CAD build for the part. Positions are in the model's coordinates, mm. Face numbers are marked on the shaded views. Round coordinates to 2 decimals unless told otherwise and drop trailing zeros. Loops run counter-clockwise (first coordinate to the right, second up) from the corner with the lowest first, then second, coordinate; pieces in that order, holes last.
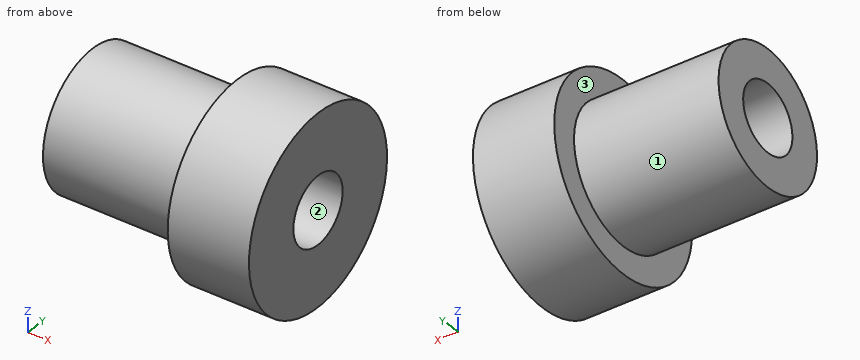
```python
from build123d import *

# Parameters (mm, degrees)
SKETCH1_R                           = 3.96875
BOSS_EXTRUDE1_DEPTH                 = 8.466666667
SKETCH2_R                           = 5.5626
BOSS_EXTRUDE2_DEPTH                 = 4.7625
F_5_32_0_15625_DIAMETER_HOLE1_D     = 3.96875
F_5_32_0_15625_DIAMETER_HOLE1_DEPTH = 70.104
F_5_32_0_15625_DIAMETER_HOLE1_TIP   = 1.192332791


with BuildPart() as part:
    # Sketch1 → Boss-Extrude1 (new body)
    with BuildSketch(Plane(origin=(0, 0, 0), x_dir=(0, 0, -1), z_dir=(1, 0, 0))):
        Circle(SKETCH1_R)
    extrude(amount=BOSS_EXTRUDE1_DEPTH)

    # Sketch2 → Boss-Extrude2 (add)
    with BuildSketch(Plane(origin=(8.466666667, 0, 0), x_dir=(0, 0, -1), z_dir=(1, 0, 0))):
        with Locations(Location((0, 0, 0), (0, 0, 180))):
            Circle(SKETCH2_R)
    extrude(amount=BOSS_EXTRUDE2_DEPTH)

    # 5/32 (0.15625) Diameter Hole1
    with Locations(Plane(origin=(13.229166667, 0, 0), x_dir=(0, 0, -1), z_dir=(1, 0, 0))):
        with Locations((0, 0)):
            Hole(F_5_32_0_15625_DIAMETER_HOLE1_D / 2, depth=F_5_32_0_15625_DIAMETER_HOLE1_DEPTH)
            with Locations((0, 0, -(F_5_32_0_15625_DIAMETER_HOLE1_DEPTH + F_5_32_0_15625_DIAMETER_HOLE1_TIP / 2))):  # 118° drill point
                Cone(0, F_5_32_0_15625_DIAMETER_HOLE1_D / 2, F_5_32_0_15625_DIAMETER_HOLE1_TIP, mode=Mode.SUBTRACT)


solid = part.part
```
Item 1: Flat gauge pins, fed straight in: P1, Ø1.5, axis at x = 8.5, y = 3, coming from the +Z side; P2, Ø1.5, axis at x = 5, y = 2.5, coming from the +Z side; P3, Ø4, axis at x = 2, y = -2.5, coming from the -Z side. Where does each tip first touch, or does it go through?
Answers follow:
P1: stops at z = 5.09
P2: stops at z = 3.56
P3: stops at z = -3.94
Item 2: Cut at C-C, the plane x = 5. Give the cut face in (y, z).
Answers follow:
outline: circle Ø7.94 at (0, 0); hole circle Ø3.97 at (0, 0)
Item 3: Probe line 1 (X direction, y = -3.5, z = 3.5); line 2 (Y direction, x = 5.5, z = 0); line 3 (Y direction, x = 8, z = 1). List the from-to ranges inside material, lowest first.
Answers follow:
line 1: x = 8.47 to 13.23
line 2: y = -3.97 to -1.98, 1.98 to 3.97
line 3: y = -3.84 to -1.71, 1.71 to 3.84
Item 4: Cut at D-D, the plane z = 2.5. Give the cut face in (x, y), plus the area to 3 significant figures.
Answers follow:
outline: (0, -3.08) - (8.47, -3.08) - (8.47, -4.97) - (13.23, -4.97) - (13.23, 4.97) - (8.47, 4.97) - (8.47, 3.08) - (0, 3.08) - close
area: 99.5 mm2
Item 5: Two-plate mould, pull along Z, no slides. Class the marked faces 1, 2 and 3: released by +Z, released by -Z, zero draft, split by the parting line, or undercut.
Answers follow:
face 1: split by the parting line
face 2: undercut
face 3: zero draft
Item 6: Cut at A-A, the plane y = 0. Give the cut face in (x, z).
Answers follow:
outline: (0, -3.97) - (8.47, -3.97) - (8.47, -5.56) - (13.23, -5.56) - (13.23, -1.98) - (0, -1.98) - close; (0, 1.98) - (13.23, 1.98) - (13.23, 5.56) - (8.47, 5.56) - (8.47, 3.97) - (0, 3.97) - close
